The listing builds one solid part. Answer for the finished solid, in the listing's coordinates (mm). A direction names the side the tool comes from. Coordinates: 2 decimals unless noted, no trailing zeros. Write each loop counter-clockwise with the first axis right and the second up, starting at its lowest first coordinate (ties: lowest second). Pieces come first, ordered by that corner, then holes. Notation, with made-up numbers: M 72,-14.5 L 115,-14.5 A5 cw 115,-6.5 Z; hole C 67,66 d11. An arc over 180 degrees is marked long. Answer as CSV lines item,"result". Start each with the question number.
```python
from build123d import *

# Parameters (mm, degrees)
SKETCH1_W           = 80
SKETCH1_H           = 59
BOSS_EXTRUDE1_DEPTH = 10.85
SKETCH2_R           = 2
CUT_EXTRUDE1_DEPTH  = 8.85
SHELL3_START        = 4.15
SHELL3_DEPTH        = 6.7
SKETCH3_R           = 1.6
CUT_EXTRUDE2_DEPTH  = 8.85
SKETCH4_W           = 10
SKETCH4_H           = 6.7
CUT_EXTRUDE3_DEPTH  = 8.85
SKETCH5_W           = 2.4
SKETCH5_H           = 18
CUT_EXTRUDE4_DEPTH  = 6.7
FILLET1_R           = 4
FILLET2_R           = 3


# Read off the part's stored shape, not the designer's step: Shell3
with BuildPart() as part:
    # Sketch1 → Boss-Extrude1 (new body)
    with BuildSketch(Plane(origin=(0, 0, 0), x_dir=(1, 0, 0), z_dir=(0, 1, 0))):
        Rectangle(SKETCH1_W, SKETCH1_H)
    extrude(amount=BOSS_EXTRUDE1_DEPTH)

    # Sketch2 → Cut-Extrude1 (cut)
    with BuildSketch(Plane(origin=(0, 10.85, 0), x_dir=(1, 0, 0), z_dir=(0, 1, 0))):
        with Locations(Location((-35.25, 24.75, 0), (0, 0, 270))):
            Circle(SKETCH2_R)
        with Locations(Location((-35.25, -24.75, 0), (0, 0, 270))):
            Circle(SKETCH2_R)
        with Locations(Location((35.25, 24.75, 0), (0, 0, 270))):
            Circle(SKETCH2_R)
        with Locations(Location((35.25, -24.75, 0), (0, 0, 270))):
            Circle(SKETCH2_R)
    extrude(amount=-CUT_EXTRUDE1_DEPTH, mode=Mode.SUBTRACT)

    # Shell3 outline → Shell3 (cut)
    with BuildSketch(Plane(origin=(0, 0, 0), x_dir=(1, 0, 0), z_dir=(0, 1, 0)).offset(SHELL3_START)):
        with BuildLine():
            ThreePointArc((-35.85, -18.629338271), (-30.901293296, -20.401293296), (-29.129338271, -25.35))
            Line((-29.129338271, -25.35), (29.129338271, -25.35))
            ThreePointArc((29.129338271, -25.35), (30.901293296, -20.401293296), (35.85, -18.629338271))
            Line((35.85, -18.629338271), (35.85, 18.629338271))
            ThreePointArc((35.85, 18.629338271), (30.901293296, 20.401293296), (29.129338271, 25.35))
            Line((29.129338271, 25.35), (-29.129338271, 25.35))
            ThreePointArc((-29.129338271, 25.35), (-30.901293296, 20.401293296), (-35.85, 18.629338271))
            Line((-35.85, 18.629338271), (-35.85, -18.629338271))
        make_face()
    extrude(amount=SHELL3_DEPTH, mode=Mode.SUBTRACT)

    # Sketch3 → Cut-Extrude2 (cut)
    with BuildSketch(Plane(origin=(0, 4.15, 0), x_dir=(1, 0, 0), z_dir=(0, 1, 0))):
        with Locations(Location((-30, -11.5, 0), (0, 0, 270))):
            Circle(SKETCH3_R)
        with Locations(Location((9, -11.5, 0), (0, 0, 270))):
            Circle(SKETCH3_R)
        with Locations(Location((9, 11.5, 0), (0, 0, 270))):
            Circle(SKETCH3_R)
        with Locations(Location((-30, 11.5, 0), (0, 0, 270))):
            Circle(SKETCH3_R)
    extrude(amount=-CUT_EXTRUDE2_DEPTH, mode=Mode.SUBTRACT)

    # Sketch4 → Cut-Extrude3 (cut)
    with BuildSketch(Plane.ZY.offset(40)):
        with Locations((0, 7.5)):
            Rectangle(SKETCH4_W, SKETCH4_H)
    extrude(amount=-CUT_EXTRUDE3_DEPTH, mode=Mode.SUBTRACT)

    # Sketch5 → Cut-Extrude4 (cut)
    with BuildSketch(Plane(origin=(0, 10.85, 0), x_dir=(1, 0, 0), z_dir=(0, 1, 0))):
        with Locations((-37.05, 0)):
            Rectangle(SKETCH5_W, SKETCH5_H)
    extrude(amount=-CUT_EXTRUDE4_DEPTH, mode=Mode.SUBTRACT)

    # Fillet1
    fillet1_edges = [part.edges().sort_by_distance(p)[0] for p in [
        (40, 5.425, 29.5),
        (-40, 5.425, 29.5),
        (-40, 5.425, -29.5),
        (40, 5.425, -29.5),
    ]]
    fillet(fillet1_edges, radius=FILLET1_R)

    # Fillet2
    # the kernel refuses this fillet: 3 mm, written as the material it takes off along each edge
    with BuildSketch(Plane(origin=(-40, 17.667945072, -5), x_dir=(0, 0, -1), z_dir=(0, -1, 0)), Plane(origin=(-40, 4.15, 5), x_dir=(0, 0, 1), z_dir=(0, 1, 0))) as fillet2_piece_1:
        with BuildLine():
            CenterArc((2.727178029, 3), FILLET2_R, 204.624318352, 65.375681648)
            Line((0, 1.75), (-0.054543561, 1.725))
            ThreePointArc((-0.054543561, 1.725), (-0.06, 0.875), (-0.06, 0))
            Line((-0.06, 0), (0, -0.06))
            Line((0, -0.06), (2.727178029, -0.06))
            Line((2.727178029, -0.06), (2.727178029, 0))
        make_face()
    extrude(amount=13.517945072, mode=Mode.SUBTRACT)
    with BuildSketch(Plane(origin=(-40, 4.15, -12.5), x_dir=(0, -1, 0), z_dir=(0, 0, 1))) as fillet2_piece_2_section:
        with BuildLine():
            CenterArc((FILLET2_R, FILLET2_R), FILLET2_R, 180, 90)
            Line((0, FILLET2_R), (-FILLET2_R * 0.02, FILLET2_R))
            Line((-FILLET2_R * 0.02, FILLET2_R), (-FILLET2_R * 0.02, -FILLET2_R * 0.02))
            Line((-FILLET2_R * 0.02, -FILLET2_R * 0.02), (FILLET2_R, -FILLET2_R * 0.02))
            Line((FILLET2_R, -FILLET2_R * 0.02), (FILLET2_R, 0))
        make_face()
    fillet2_piece_2 = extrude(amount=17.5, mode=Mode.PRIVATE)
    fillet2_piece_2 = split(fillet2_piece_2, bisect_by=Plane(origin=(-37.813587666, 4.113532684, -5), z_dir=(0, 0, -1)), keep=Keep.TOP, mode=Mode.PRIVATE)
    fillet2_piece_2 = split(fillet2_piece_2, bisect_by=Plane(origin=(-38.25, 4.113532684, -7), z_dir=(1, 0, 0)), keep=Keep.TOP, mode=Mode.PRIVATE)
    fillet2_piece_2 = split(fillet2_piece_2, bisect_by=Plane(origin=(-37.813587666, 4.113532684, -9), z_dir=(0, 0, 1)), keep=Keep.TOP, mode=Mode.PRIVATE)
    add(fillet2_piece_2, mode=Mode.SUBTRACT)
    with BuildSketch(Plane(origin=(-40, 4.15, -5), x_dir=(0, -1, 0), z_dir=(0, 0, 1))) as fillet2_piece_3_section:
        with BuildLine():
            CenterArc((FILLET2_R, FILLET2_R), FILLET2_R, 180, 90)
            Line((0, FILLET2_R), (-FILLET2_R * 0.02, FILLET2_R))
            Line((-FILLET2_R * 0.02, FILLET2_R), (-FILLET2_R * 0.02, -FILLET2_R * 0.02))
            Line((-FILLET2_R * 0.02, -FILLET2_R * 0.02), (FILLET2_R, -FILLET2_R * 0.02))
            Line((FILLET2_R, -FILLET2_R * 0.02), (FILLET2_R, 0))
        make_face()
    fillet2_piece_3 = extrude(amount=10, mode=Mode.PRIVATE)
    fillet2_piece_3 = split(fillet2_piece_3, bisect_by=Plane(origin=(-38.25, 3.413957666, 0), z_dir=(-1, 0, 0)), keep=Keep.TOP, mode=Mode.PRIVATE)
    add(fillet2_piece_3, mode=Mode.SUBTRACT)
    with BuildSketch(Plane(origin=(-40, 4.15, -5), x_dir=(0, -1, 0), z_dir=(0, 0, 1))) as fillet2_piece_4_section:
        with BuildLine():
            CenterArc((FILLET2_R, FILLET2_R), FILLET2_R, 180, 90)
            Line((0, FILLET2_R), (-FILLET2_R * 0.02, FILLET2_R))
            Line((-FILLET2_R * 0.02, FILLET2_R), (-FILLET2_R * 0.02, -FILLET2_R * 0.02))
            Line((-FILLET2_R * 0.02, -FILLET2_R * 0.02), (FILLET2_R, -FILLET2_R * 0.02))
            Line((FILLET2_R, -FILLET2_R * 0.02), (FILLET2_R, 0))
        make_face()
    fillet2_piece_4 = extrude(amount=10, mode=Mode.PRIVATE)
    fillet2_piece_4 = split(fillet2_piece_4, bisect_by=Plane(origin=(-38.25, 4.113532684, 0), z_dir=(1, 0, 0)), keep=Keep.TOP, mode=Mode.PRIVATE)
    add(fillet2_piece_4, mode=Mode.SUBTRACT)
    with BuildSketch(Plane(origin=(-40, 4.15, -5), x_dir=(0, -1, 0), z_dir=(0, 0, 1))) as fillet2_piece_5_section:
        with BuildLine():
            CenterArc((FILLET2_R, FILLET2_R), FILLET2_R, 180, 90)
            Line((0, FILLET2_R), (-FILLET2_R * 0.02, FILLET2_R))
            Line((-FILLET2_R * 0.02, FILLET2_R), (-FILLET2_R * 0.02, -FILLET2_R * 0.02))
            Line((-FILLET2_R * 0.02, -FILLET2_R * 0.02), (FILLET2_R, -FILLET2_R * 0.02))
            Line((FILLET2_R, -FILLET2_R * 0.02), (FILLET2_R, 0))
        make_face()
    fillet2_piece_5 = extrude(amount=17.5, mode=Mode.PRIVATE)
    fillet2_piece_5 = split(fillet2_piece_5, bisect_by=Plane(origin=(-38.25, 4.113532684, 7), z_dir=(1, 0, 0)), keep=Keep.TOP, mode=Mode.PRIVATE)
    fillet2_piece_5 = split(fillet2_piece_5, bisect_by=Plane(origin=(-37.813587666, 4.113532684, 5), z_dir=(0, 0, 1)), keep=Keep.TOP, mode=Mode.PRIVATE)
    fillet2_piece_5 = split(fillet2_piece_5, bisect_by=Plane(origin=(-37.813587666, 4.113532684, 9), z_dir=(0, 0, -1)), keep=Keep.TOP, mode=Mode.PRIVATE)
    add(fillet2_piece_5, mode=Mode.SUBTRACT)
    with BuildSketch(Plane(origin=(-40, 17.667945072, -5), x_dir=(0, 0, -1), z_dir=(0, -1, 0))) as fillet2_piece_6a_section:
        with BuildLine():
            CenterArc((2.727178029, 3), FILLET2_R, 204.624318352, 65.375681648)
            Line((0, 1.75), (-0.054543561, 1.725))
            ThreePointArc((-0.054543561, 1.725), (-0.06, 0.875), (-0.06, 0))
            Line((-0.06, 0), (0, -0.06))
            Line((0, -0.06), (2.727178029, -0.06))
            Line((2.727178029, -0.06), (2.727178029, 0))
        make_face()
    fillet2_piece_6a = extrude(amount=20.335890143, mode=Mode.PRIVATE)
    fillet2_piece_6a = split(fillet2_piece_6a, bisect_by=Plane(origin=(-39.546962739, 4.15, -5.666780032), z_dir=(0, -1, 0)), keep=Keep.TOP, mode=Mode.PRIVATE)
    with BuildSketch(Plane(origin=(-40, 4.15, -12.5), x_dir=(0, -1, 0), z_dir=(0, 0, 1))) as fillet2_piece_6b_section:
        with BuildLine():
            CenterArc((FILLET2_R, FILLET2_R), FILLET2_R, 180, 90)
            Line((0, FILLET2_R), (-FILLET2_R * 0.02, FILLET2_R))
            Line((-FILLET2_R * 0.02, FILLET2_R), (-FILLET2_R * 0.02, -FILLET2_R * 0.02))
            Line((-FILLET2_R * 0.02, -FILLET2_R * 0.02), (FILLET2_R, -FILLET2_R * 0.02))
            Line((FILLET2_R, -FILLET2_R * 0.02), (FILLET2_R, 0))
        make_face()
    fillet2_piece_6b = extrude(amount=17.5, mode=Mode.PRIVATE)
    fillet2_piece_6b = split(fillet2_piece_6b, bisect_by=Plane(origin=(-39.454149009, 3.413957666, -5), z_dir=(0, 0, -1)), keep=Keep.TOP, mode=Mode.PRIVATE)
    fillet2_piece_6b = split(fillet2_piece_6b, bisect_by=Plane(origin=(-38.25, 3.413957666, -7), z_dir=(-1, 0, 0)), keep=Keep.TOP, mode=Mode.PRIVATE)
    fillet2_piece_6b = split(fillet2_piece_6b, bisect_by=Plane(origin=(-39.454149009, 3.413957666, -9), z_dir=(0, 0, 1)), keep=Keep.TOP, mode=Mode.PRIVATE)
    fillet2_piece_6 = fillet2_piece_6a & fillet2_piece_6b
    add(fillet2_piece_6, mode=Mode.SUBTRACT)
    with BuildSketch(Plane(origin=(-40, -2.667945072, 5), x_dir=(0, 0, 1), z_dir=(0, 1, 0))) as fillet2_piece_7a_section:
        with BuildLine():
            CenterArc((2.727178029, 3), FILLET2_R, 204.624318352, 65.375681648)
            Line((0, 1.75), (-0.054543561, 1.725))
            ThreePointArc((-0.054543561, 1.725), (-0.06, 0.875), (-0.06, 0))
            Line((-0.06, 0), (0, -0.06))
            Line((0, -0.06), (2.727178029, -0.06))
            Line((2.727178029, -0.06), (2.727178029, 0))
        make_face()
    fillet2_piece_7a = extrude(amount=20.335890143, mode=Mode.PRIVATE)
    fillet2_piece_7a = split(fillet2_piece_7a, bisect_by=Plane(origin=(-39.546962739, 4.15, 5.666780032), z_dir=(0, -1, 0)), keep=Keep.TOP, mode=Mode.PRIVATE)
    with BuildSketch(Plane(origin=(-40, 4.15, -5), x_dir=(0, -1, 0), z_dir=(0, 0, 1))) as fillet2_piece_7b_section:
        with BuildLine():
            CenterArc((FILLET2_R, FILLET2_R), FILLET2_R, 180, 90)
            Line((0, FILLET2_R), (-FILLET2_R * 0.02, FILLET2_R))
            Line((-FILLET2_R * 0.02, FILLET2_R), (-FILLET2_R * 0.02, -FILLET2_R * 0.02))
            Line((-FILLET2_R * 0.02, -FILLET2_R * 0.02), (FILLET2_R, -FILLET2_R * 0.02))
            Line((FILLET2_R, -FILLET2_R * 0.02), (FILLET2_R, 0))
        make_face()
    fillet2_piece_7b = extrude(amount=17.5, mode=Mode.PRIVATE)
    fillet2_piece_7b = split(fillet2_piece_7b, bisect_by=Plane(origin=(-38.25, 3.413957666, 7), z_dir=(-1, 0, 0)), keep=Keep.TOP, mode=Mode.PRIVATE)
    fillet2_piece_7b = split(fillet2_piece_7b, bisect_by=Plane(origin=(-39.454149009, 3.413957666, 5), z_dir=(0, 0, 1)), keep=Keep.TOP, mode=Mode.PRIVATE)
    fillet2_piece_7b = split(fillet2_piece_7b, bisect_by=Plane(origin=(-39.454149009, 3.413957666, 9), z_dir=(0, 0, -1)), keep=Keep.TOP, mode=Mode.PRIVATE)
    fillet2_piece_7 = fillet2_piece_7a & fillet2_piece_7b
    add(fillet2_piece_7, mode=Mode.SUBTRACT)


solid = part.part
```
1) Each of these flat-tipped pins is pushed along its axis until it touches: P1, Ø2, axis at x = 34.5, z = 24.5, coming from the +Y side; P2, Ø15, axis at x = -18, z = 8.5, coming from the +Y side. Where does it stop, or does it pass through?
2) Which of the six approach directions +Z, -Z, +X, -X, +Y, -Y give full straight-line access (tool end or side, diameter ignored) to faces 5 (the face through (8.03, 2.1, -12.77)), 6 (the face through (-38.25, 7, -7))?
3) The part is cut by section A-A (x = 9). Determine the outline of the cut face in (y, z), then the cut area to 3 significant figures.
4) The part is cut by section B-B (z = -11.5). Determine the outline of the cut face in (x, y), then the cut area to 3 significant figures.
5) The part is cut by section C-C (x = -22). Determine the outline of the cut face in (y, z).
6) For a pull along X with two mould halves and no side action, classify faces 1 (the face through (0, 7, 25.35)), 2 (the face through (-1, 5, 29.5)), 3 (the face through (-28.92, 2.1, 10.32)), 4 (the face through (-38.859, 5.501, 28.297)) as +X half, -X half, draft (parallel to the pull), parting line (faces both ways), or undercut.
7) Find the intervals of material crossed by line 1 (X direction, y = 2.3, z = 11.5); line 2 (X direction, y = 8, z = -24.75); line 3 (Z direction, x = -11, y = 10), in increasing order. Write a range as from..to.
Completed:
1,P1,"y = 2"
1,P2,"y = 4.15"
2,face 5,"+Y, -Y"
2,face 6,"+Y"
3,outline,"M 0,-29.5 L 10.85,-29.5 L 10.85,-25.35 L 4.15,-25.35 L 4.15,-13.1 L 0,-13.1 Z; M 0,-9.9 L 4.15,-9.9 L 4.15,9.9 L 0,9.9 Z; M 0,13.1 L 4.15,13.1 L 4.15,25.35 L 10.85,25.35 L 10.85,29.5 L 0,29.5 Z"
3,area,"274 mm²"
4,outline,"M -40,0 L -31.6,0 L -31.6,4.15 L -35.85,4.15 L -35.85,10.85 L -40,10.85 Z; M -28.4,0 L 7.4,0 L 7.4,4.15 L -28.4,4.15 Z; M 10.6,0 L 40,0 L 40,10.85 L 35.85,10.85 L 35.85,4.15 L 10.6,4.15 Z"
4,area,"361 mm²"
5,outline,"M 0,-29.5 L 10.85,-29.5 L 10.85,-25.35 L 4.15,-25.35 L 4.15,25.35 L 10.85,25.35 L 10.85,29.5 L 0,29.5 Z"
6,face 1,"undercut"
6,face 2,"draft"
6,face 3,"undercut"
6,face 4,"-X half"
7,line 1,"-40..-31.6, -28.4..7.4, 10.6..40"
7,line 2,"-40..-37.25, -33.25..-29.1, 29.1..33.25, 37.25..40"
7,line 3,"-29.5..-25.35, 25.35..29.5"
